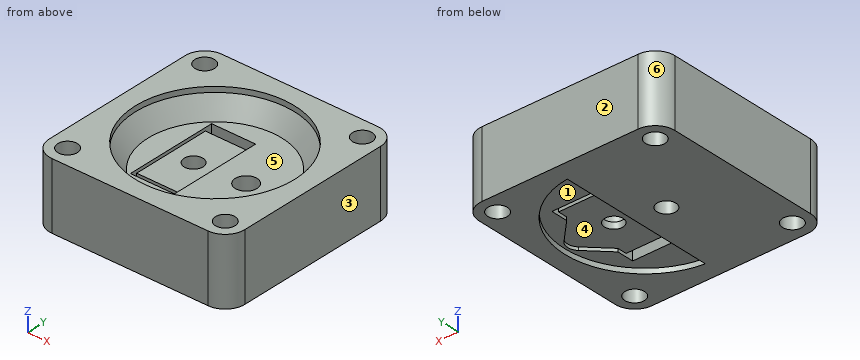
```python
from build123d import *

# Parameters (mm, degrees)
F1_DEPTH        = 10.795
F5_D            = 3.175
F5_COPIES_COUNT = 4
F7_D            = 2.9972
F7_CBORE_D      = 3.5306
F7_CBORE_DEPTH  = 4.6228
F9_D            = 3.048
F10_W           = 7.112
F10_H           = 15.113
F11_DEPTH       = 0.508
F12_W           = 7.112
F12_H           = 1.1684
F13_DEPTH       = 2.159
F15_DEPTH       = 0.8128
F16_W           = 7.112
F16_H           = 15.0114
F17_DEPTH       = 0.508
F18_W           = 7.112
F18_H           = 1.2192
F19_DEPTH       = 2.159
F21_DEPTH       = 0.508


# Not quite as in the source:
# - a pattern or mirror of a feature is missing from the dataset's text; its kind, count and spacing are read off the source's solid


with BuildPart() as f1:
    # F0 (on Top) → F1 (new body)
    with BuildSketch(Plane.XY):
        with BuildLine():
            Line((12.6365, 15.8115), (-12.6365, 15.8115))
            ThreePointArc((-12.6365, 15.8115), (-14.8815640303, 14.8815640303), (-15.8115, 12.6365))
            Line((-15.8115, 12.6365), (-15.8115, -12.6365))
            ThreePointArc((-15.8115, -12.6365), (-14.8815640303, -14.8815640303), (-12.6365, -15.8115))
            Line((-12.6365, -15.8115), (12.6365, -15.8115))
            ThreePointArc((12.6365, -15.8115), (14.8815640303, -14.8815640303), (15.8115, -12.6365))
            Line((15.8115, -12.6365), (15.8115, 12.6365))
            ThreePointArc((15.8115, 12.6365), (14.8815640303, 14.8815640303), (12.6365, 15.8115))
        make_face()
    extrude(amount=F1_DEPTH)

    # F2 (on Front) → F3 (revolve, cut)
    with BuildSketch(Plane.XZ):
        Polygon((0, 10.795), (0, 6.985), (10.8204, 6.985), (12.8651, 9.9314), (12.8651, 10.795), align=None)
    revolve(axis=Axis((0, 0, 1.5018361828), (0, 0, -1)), mode=Mode.SUBTRACT)

    # F5 (through all)
    with Locations(Plane.XY.offset(10.795)):
        with Locations((-12.7519636919, 12.7519636919)):
            f5 = Hole(F5_D / 2)

    # F5_copies: F5 ×4 about axis
    f5_copies_axis = Axis((0, 0, 0), (0, 0, 1))
    for i in range(1, F5_COPIES_COUNT):
        add(f5.rotate(f5_copies_axis, i * 360 / F5_COPIES_COUNT), mode=Mode.SUBTRACT)

    # F7 (through all)
    with Locations(Plane.XY.offset(6.985)):
        with Locations((5.0419, 0)):
            CounterBoreHole(F7_D / 2, F7_CBORE_D / 2, F7_CBORE_DEPTH)

    # F9 (through all)
    with Locations(Plane.XY.offset(6.985)):
        with Locations((-3.4671, 0)):
            Hole(F9_D / 2)

    # F10 (on face) → F11 (cut)
    with BuildSketch(Plane.XY.offset(6.985)):
        with Locations((-3.556, 0)):
            Rectangle(F10_W, F10_H)
    extrude(amount=-F11_DEPTH, mode=Mode.SUBTRACT)

    # F12 (on face) → F13 (cut)
    with BuildSketch(Plane.XY.offset(6.985)):
        with Locations((-3.556, 6.9723)):
            Rectangle(F12_W, F12_H)
    f13 = extrude(amount=-F13_DEPTH, mode=Mode.SUBTRACT)

    # F13_copies: F13 across plane
    add(f13.mirror(Plane(origin=(0, 0, 0), x_dir=(0, 0, -1), z_dir=(0, -1, 0))), mode=Mode.SUBTRACT)

    # F14 (on face) → F15 (cut)
    with BuildSketch(Plane(origin=(0, 0, 0), x_dir=(1, 0, 0), z_dir=(0, 0, -1))):
        with BuildLine():
            ThreePointArc((1.4097, -12.8524), (12.9413, 0), (1.4097, 12.8524))
            Line((1.4097, 12.8524), (1.4097, -12.8524))
        make_face()
    extrude(amount=-F15_DEPTH, mode=Mode.SUBTRACT)

    # F16 (on face) → F17 (cut)
    with BuildSketch(Plane(origin=(0, 0, 0.8128), x_dir=(1, 0, 0), z_dir=(0, 0, -1))):
        with Locations((4.9657, 0)):
            Rectangle(F16_W, F16_H)
    extrude(amount=-F17_DEPTH, mode=Mode.SUBTRACT)

    # F18 (on face) → F19 (cut)
    with BuildSketch(Plane(origin=(0, 0, 0.8128), x_dir=(1, 0, 0), z_dir=(0, 0, -1))):
        with Locations((4.9657, 6.8961)):
            Rectangle(F18_W, F18_H)
    f19 = extrude(amount=-F19_DEPTH, mode=Mode.SUBTRACT)

    # F19_copies: F19 across plane
    add(f19.mirror(Plane.ZX), mode=Mode.SUBTRACT)

    # F20 (on face) → F21 (cut, through all)
    with BuildSketch(Plane(origin=(0, 0, 0.8128), x_dir=(1, 0, 0), z_dir=(0, 0, -1))):
        with BuildLine():
            Line((11.9371615818, 1.3470384182), (8.5217, 4.7625))
            Line((8.5217, 4.7625), (8.5217, -4.7625))
            Line((8.5217, -4.7625), (11.9371615818, -1.3470384182))
            ThreePointArc((11.9371615818, -1.3470384182), (12.4951231637, 0), (11.9371615818, 1.3470384182))
        make_face()
    extrude(amount=-F21_DEPTH, mode=Mode.SUBTRACT)


solid = f1.part
```
Read the model definition and answer for the solid it produces. Units are mm, in the model's axes. Face numbers are marked on the shaded views. A direction names the side the tool comes from. Coordinates: 2 decimals unless noted, no trailing zeros. Answer as a JSON object with one key per item and string values.
Q1. The part is cut by section A-A on y = 0. Give the number of separate pieces and of enclosed holes in the cut face, then the cut area to 3 significant figures.
The answers:
{"separate pieces": "3", "enclosed holes": "0", "area": "192 mm2"}
Q2. Flat-ended cylindrical pins translate along their axes: pin 1 Ø0.9 at (x, y) = (-5, 7) entering from +Z; pin 2 Ø1 at (x, y) = (4.5, 8) entering from -Z; pin 3 Ø4.5 at (x, y) = (5.04, 0) entering from -Z; pin 4 Ø2.5 at (x, y) = (-3.47, 0) entering from -Z. Find the tip coordinate at first contact, or state that the pin passes through.
The answers:
{"pin 1": "stops at z = 4.83", "pin 2": "stops at z = 0.81", "pin 3": "stops at z = 1.32", "pin 4": "passes through"}
Q3. Consider line 1 (Y direction, x = 2, z = 2); line 2 (Y direction, x = -6.5, z = 6); line 3 (X direction, y = 0, z = 10.5). Determine where each line is inside the solid, lowest interval first. Write a range as [from, to].
The answers:
{"line 1": "y = [-15.81, -7.51], [-6.29, 6.29], [7.51, 15.81]", "line 2": "y = [-15.81, -7.56], [-6.39, 6.39], [7.56, 15.81]", "line 3": "x = [-15.81, -12.87], [12.87, 15.81]"}
Q4. Determine the mould class of the marked faces 1, 2 and 3 for opening direction X: pulls with the +X half, pulls with the -X half, needs draft (parallel to the pull), parting line crosses it, or undercut.
The answers:
{"face 1": "undercut", "face 2": "needs draft", "face 3": "pulls with the +X half"}
Q5. A tool of negligible diameter and unlimited length cuts with its end or side. For the marked faces 4, 5 and 6, from which of +Z, -Z, +X, -X, +Y, -Y can it reach the whole face along a straight path? Write none if from no direction.
The answers:
{"face 4": "-Z", "face 5": "+Z", "face 6": "+Z, -Z, -X, +Y"}
